Drawing for the job (mm, zero at the part's lowest x, y, z). A direction names the side the tool comes from. Give positions to 0.01 mm unless a question says otherwise; leave off trailing zeros. Loops run counter-clockwise (first coordinate to the right, second up) from the corner with the lowest first, then second, coordinate; pieces in that order, holes last. Notation, with made-up numbers: (-28.75, 19) - (-14.75, 19) arc R21 cw to (-14.75, 42) - close; hole circle Ø10 at (76.5, 86.25). An arc over 180 degrees is marked (long way). Return JSON: item names as keys, results as strings. Group by question number.
1) Mould opens along Y. For the marked faces 1, 2 and 3 say: released by +Y, released by -Y, zero draft, split by the parting line, or undercut.
2) 3-axis set-ups, long thin cutter, end or side, ignore diameter. For the marked faces 4 and 5: which of +Z, -Z, +X, -X, +Y, -Y reach the whole face in a straight line?
3) Drop flat-ended pins along their axis: pin 1 (6 mm diameter, centred on y = 7, z = 6, fed in from +X) (1 decimal); pin 2 (3.5 mm diameter, centred on x = 13.5, y = 13, fed in from +Z); pin 3 (2.5 mm diameter, centred on x = 13, y = 13, fed in from +Z); pin 4 (4 mm diameter, centred on x = 13.5, y = 6, fed in from +Z). Give the stop position or say it passes through.
4) Slice it at B-B (z = 5.5). List the corners of the cut face in (x, y).
5) Slice it at C-C (z = 8.5). List the corners of the cut face in (x, y).
6) Drill centre lines: probe 1 along Y at (x, z) = (13, 2); probe 2 along Z at (x, y) = (8.75, 14); probe 3 along Y at (x, z) = (11.75, 1.75) (1 decimal). Where is each one in solid material? Low to high. Write a range as from..to.
7) Slice it at A-A (x = 13). Count the separate pieces of the cut face and the enclosed holes in it.
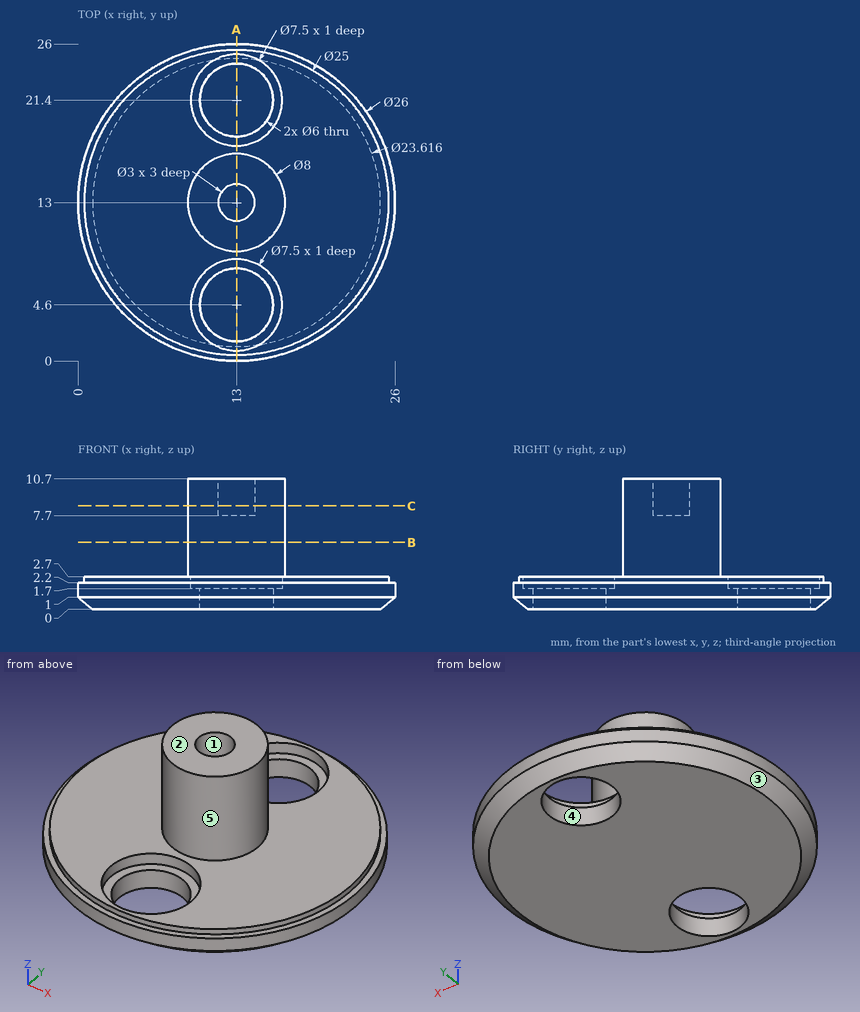
Results:
{
 "1": {"face 1": "undercut", "face 2": "zero draft", "face 3": "split by the parting line"},
 "2": {"face 4": "+Z, -Z", "face 5": "+Z"},
 "3": {"pin 1": "x = 15.6", "pin 2": "z = 10.7", "pin 3": "z = 7.7", "pin 4": "z = 1.7"},
 "4": {"outline": "circle Ø8 at (13, 13)"},
 "5": {"outline": "circle Ø8 at (13, 13); hole circle Ø3 at (13, 13)"},
 "6": {"probe 1": "0..0.85, 8.35..17.65, 25.15..26", "probe 2": "0..2.7", "probe 3": "0.1..1.1, 8.1..17.9, 24.9..25.9"},
 "7": {"separate pieces": "3", "enclosed holes": "0"}
}
